Autodesk Inventor part; units mm, degrees
ref_plane "YZ Plane" through (0, 0, 0) normal (1, 0, 0) x (0, 1, 0)
ref_plane "XZ Plane" through (0, 0, 0) normal (0, 1, 0) x (-1, 0, 0)
ref_plane "XY Plane" through (0, 0, 0) normal (0, 0, 1) x (1, 0, 0)
sketch "Sketch1" plane through (0, 0, 0) normal (1, 0, 0) x (0, 1, 0)
  line L0 (11, 31.5) -> (-11, 31.5)
  line L1 (-11, 31.5) -> (-11, -31.5)
  line L2 (-11, -31.5) -> (11, -31.5)
  line L3 (11, -31.5) -> (11, 31.5)
  line L4 (11, 31.5) -> (-11, -31.5) construction
  line L5 (-11, 31.5) -> (11, -31.5) construction
  point P0 (0, 0)
  dimension "d0" = 22
  dimension "d1" = 63
extrude "Extrusion1" add sketch "Sketch1" along normal mid plane 141
fillet "Fillet1" radius 6 4 edges at (0, 11, 31.5) (0, 11, -31.5) (0, -11, 31.5) (0, -11, -31.5)
sketch "Sketch2" plane through (70.5, 0, 0) normal (1, 0, 0) x (0, 0, -1)
  line L0 (10.5, 7) -> (24.5, 7)
  line L1 (24.5, 7) -> (24.5, 1)
  line L2 (24.5, 1) -> (10.5, 1)
  line L3 (10.5, 1) -> (10.5, 7)
  line L4 (31.5, -5) -> (31.5, 5)
  line L5 (25.5, 11) -> (-25.5, 11)
  line L6 (11.7, 5.85) -> (23.3, 5.85)
  line L7 (23.3, 5.85) -> (23.3, 4.6)
  line L8 (23.3, 4.6) -> (11.7, 4.6)
  line L9 (11.7, 4.6) -> (11.7, 5.85)
  line L10 (10.5, -2.5) -> (24.5, -2.5)
  line L11 (24.5, -2.5) -> (24.5, -8.5)
  line L12 (24.5, -8.5) -> (10.5, -8.5)
  line L13 (10.5, -8.5) -> (10.5, -2.5)
  line L14 (11.7, -3.65) -> (23.3, -3.65)
  line L15 (23.3, -3.65) -> (23.3, -4.9)
  line L16 (23.3, -4.9) -> (11.7, -4.9)
  line L17 (11.7, -4.9) -> (11.7, -3.65)
  point P0 (0, 0)
  dimension "d5" = 14
  dimension "d6" = 6
  dimension "d7" = 7
  dimension "d8" = 4
  dimension "d12" = 1.2
  dimension "d13" = 1.2
  dimension "d14" = 1.15
  dimension "d15" = 3.6
  dimension "d16" = 14
  dimension "d17" = 6
  dimension "d18" = 1.2
  dimension "d19" = 1.2
  dimension "d20" = 1.15
  dimension "d21" = 3.6
  dimension "d22" = 3.5
extrude "Extrusion2" cut sketch "Sketch2" against normal blind 10
sketch "Sketch3" plane through (-70.5, 11, -25.5) normal (0, 1, 0) x (1, 0, 0)
  line L0 (110.1613, -6.5149) -> (123.1613, -6.5149)
  line L1 (123.1613, -6.5149) -> (123.1613, -10.5149)
  line L2 (123.1613, -10.5149) -> (110.1613, -10.5149)
  line L3 (110.1613, -10.5149) -> (110.1613, -6.5149)
  line L4 (110.6613, -7.0149) -> (112.6613, -7.0149)
  line L5 (112.6613, -7.0149) -> (112.6613, -10.0149)
  line L6 (112.6613, -10.0149) -> (110.6613, -10.0149)
  line L7 (110.6613, -10.0149) -> (110.6613, -7.0149)
  line L8 (115.9613, -10.0149) -> (113.9613, -10.0149)
  line L9 (113.9613, -10.0149) -> (113.9613, -7.0149)
  line L10 (113.9613, -7.0149) -> (115.9613, -7.0149)
  line L11 (115.9613, -7.0149) -> (115.9613, -10.0149)
  line L12 (119.2613, -10.0149) -> (117.2613, -10.0149)
  line L13 (117.2613, -10.0149) -> (117.2613, -7.0149)
  line L14 (117.2613, -7.0149) -> (119.2613, -7.0149)
  line L15 (119.2613, -7.0149) -> (119.2613, -10.0149)
  line L16 (122.5613, -10.0149) -> (120.5613, -10.0149)
  line L17 (120.5613, -10.0149) -> (120.5613, -7.0149)
  line L18 (120.5613, -7.0149) -> (122.5613, -7.0149)
  line L19 (122.5613, -7.0149) -> (122.5613, -10.0149)
  point P0 (70.5, -25.5)
  dimension "d25" = 13
  dimension "d26" = 4
  dimension "d27" = 2
  dimension "d28" = 3
  dimension "d29" = 0.5
  dimension "d30" = 0.5
  dimension "d33" = 3.3
extrude "Extrusion3" cut sketch "Sketch3" against normal blind 0.25
sketch "Sketch4" plane through (70.5, -5, -31.5) normal (0, 0, -1) x (-1, 0, 0)
  line L0 (141, 10) -> (0, 10) construction
  line L1 (0, 0) -> (0, 10) construction
  line L2 (35, 5) -> (42, 5)
  line L3 (42, 5) -> (42, 8)
  line L4 (42, 8) -> (35, 8)
  line L5 (35, 8) -> (35, 5)
  line L6 (38.5, 5) -> (38.5, 8) construction
  line L7 (35, 6.5) -> (36.7876, 5)
  line L8 (35, 6.5) -> (37.3336, 6.5) construction
  line L9 (42, 6.5) -> (40.2124, 5)
  line L10 (42, 6.5) -> (42, 5)
  line L11 (40.2124, 5) -> (42, 5)
  point P0 (70.5, 5)
  dimension "d42" = 3
  dimension "d43" = 35
  dimension "d44" = 7
  dimension "d45" = 2
  dimension "d46" = 40
extrude "Extrusion4" cut sketch "Sketch4" against normal blind 5 contours L7 L5 L4 L3 L9 L2
sketch "Sketch5" plane through (70.5, -5, -31.5) normal (0, 0, -1) x (-1, 0, 0)
  line L0 (0, 0) -> (0, 10) construction
  line L1 (0, 5) -> (141, 5) construction
  line L2 (141, 10) -> (141, 0) construction
  line L3 (13, 9) -> (27, 9)
  line L4 (27, 9) -> (27, 1)
  line L5 (27, 1) -> (13, 1)
  line L6 (13, 1) -> (13, 9)
  line L7 (13, 9) -> (27, 1) construction
  line L8 (27, 9) -> (13, 1) construction
  line L9 (26.75, 8.75) -> (13.25, 8.75)
  line L10 (13.25, 8.75) -> (13.25, 1.25)
  line L11 (13.25, 1.25) -> (26.75, 1.25)
  line L12 (26.75, 1.25) -> (26.75, 8.75)
  line L13 (35, 6.5) -> (35, 8)
  point P0 (70.5, 5)
  point P1 (20, 5)
  dimension "d49" = 14
  dimension "d50" = 8
  dimension "d51" = 0.25
  dimension "d52" = 8
extrude "Extrusion5" cut sketch "Sketch5" against normal blind 0.1
sketch "Sketch6" plane through (70.5, 0, 0) normal (1, 0, 0) x (0, 0, -1)
  line L0 (10.5, 1) -> (10.5, 7)
  line L1 (10.5, 7) -> (24.5, 7)
  line L2 (24.5, 7) -> (24.5, 1)
  line L3 (24.5, 1) -> (10.5, 1)
  line L4 (10.5, -8.5) -> (10.5, -2.5)
  line L5 (10.5, -2.5) -> (24.5, -2.5)
  line L6 (24.5, -2.5) -> (24.5, -8.5)
  line L7 (24.5, -8.5) -> (10.5, -8.5)
  arc A0 (25.5, -11) -> (31.5, -5) centre (25.5, -5) ccw
  line L8 (31.5, -5) -> (31.5, 5)
  arc A1 (31.5, 5) -> (25.5, 11) centre (25.5, 5) ccw
  line L9 (25.5, 11) -> (-25.5, 11)
  arc A2 (-25.5, 11) -> (-31.5, 5) centre (-25.5, 5) ccw
  line L10 (-31.5, 5) -> (-31.5, -5)
  arc A3 (-31.5, -5) -> (-25.5, -11) centre (-25.5, -5) ccw
  line L11 (-25.5, -11) -> (25.5, -11)
  line L12 (-25.5, 10) -> (25.5, 10)
  arc A4 (30.5, 5) -> (25.5, 10) centre (25.5, 5) ccw
  line L13 (30.5, 5) -> (30.5, -5)
  arc A5 (25.5, -10) -> (30.5, -5) centre (25.5, -5) ccw
  line L14 (25.5, -10) -> (-25.5, -10)
  arc A6 (-30.5, -5) -> (-25.5, -10) centre (-25.5, -5) ccw
  line L15 (-30.5, -5) -> (-30.5, 5)
  arc A7 (-25.5, 10) -> (-30.5, 5) centre (-25.5, 5) ccw
  line L16 (-25.5, 9.75) -> (25.5, 9.75)
  arc A8 (30.25, 5) -> (25.5, 9.75) centre (25.5, 5) ccw
  line L17 (30.25, 5) -> (30.25, -5)
  arc A9 (25.5, -9.75) -> (30.25, -5) centre (25.5, -5) ccw
  line L18 (25.5, -9.75) -> (-25.5, -9.75)
  arc A10 (-30.25, -5) -> (-25.5, -9.75) centre (-25.5, -5) ccw
  line L19 (-30.25, -5) -> (-30.25, 5)
  arc A11 (-25.5, 9.75) -> (-30.25, 5) centre (-25.5, 5) ccw
  point P0 (0, 0)
  dimension "d55" = 1
  dimension "d56" = 1.25
extrude "Extrusion6" cut sketch "Sketch6" against normal blind 0.1 contours L12 A4 L13 A5 L14 A6 L15 A7
mirror "Mirror1" about plane through (0, 0, 0) normal (1, 0, 0) of "Extrusion6"
properties part number "Battery"
Design review of the part built by this model. Coordinates are the model's own, in mm. A direction names the side the tool comes from. Give positions to 0.01 mm unless a question says otherwise; leave off trailing zeros. Order: outer loops, then holes, each group sorted by start corner. A loop starts at its lowest first (then second) coordinate and runs counter-clockwise, first axis right, second up. Notation, with made-up numbers: (-28, 57) -> (27, 57) arc R19 cw to (27, 67) -> close; hole circle Ø7 at (-29, 19). An arc over 180 degrees is marked (long way). Write item = value, one per line. Start each with the question number.
(1) To check wall thickness, follow line 1 along X through (y, z) = (-7.5, -13); line 2 along Y through (x, z) = (-39, 28); line 3 along Z through (x, y) = (57.5, 8.75). State the ranges of each line that lie inside material, in increasing order.
(2) We need section B-B on y = 8.5. Write out the cut boundary in (x, z), plus the area to 3 significant figures.
(3) For faces 4 (the face through (66, -2.5, -17)), 5 (the face through (50, 0, -31.5)), list the 3-axis set-ups (+Z, -Z, +X, -X, +Y, -Y) from which the entire face can be reached by the end or side of a thin tool; tool diameter is ignored.
(4) We need section A-A on x = -25. Write out the cut boundary in (y, z).
(5) Mouldability with a two-part tool opening along Z and no side actions: class faces 1 (the face through (66, 4.6, -18)), 2 (the face through (32, 2, -26.5)), 3 (the face through (70.5, 0, 0)) as +Z half, -Z half, draft (parallel to the pull), parting line (faces both ways), or undercut.
(6) For pin 1 (3.5 mm diameter, centred on x = 30.5, y = 1.5, fed in from -Z); pin 2 (5.5 mm diameter, centred on x = 32, z = -29, fed in from -Y), all flat-tipped, find the tip position at first contact; note any pin that passes through.
Numbers:
q1.line_1 = -70.5 to 60.5
q1.line_2 = -10.45 to 10.45
q1.line_3 = -30.18 to 30.18
q2.outline = (-70.5, -30.37) -> (70.5, -30.37) -> (70.5, -29.07) -> (70.4, -29.07) -> (70.4, -28.71) -> (70.5, -28.71) -> (70.5, 28.71) -> (70.4, 28.71) -> (70.4, 29.07) -> (70.5, 29.07) -> (70.5, 30.37) -> (-70.5, 30.37) -> (-70.5, 29.07) -> (-70.4, 29.07) -> (-70.4, 28.71) -> (-70.5, 28.71) -> (-70.5, -28.71) -> (-70.4, -28.71) -> (-70.4, -29.07) -> (-70.5, -29.07) -> close
q2.area = 8,570 mm^2
q3.face_4 = +X
q3.face_5 = -Z, +X, -X, +Y, -Y
q4.outline = (-11, -25.5) arc R6 ccw to (-5, -31.5) -> (5, -31.5) arc R6 ccw to (11, -25.5) -> (11, 25.5) arc R6 ccw to (5, 31.5) -> (-5, 31.5) arc R6 ccw to (-11, 25.5) -> close
q5.face_1 = undercut
q5.face_2 = -Z half
q5.face_3 = draft
q6.pin_1 = -31.5
q6.pin_2 = -10.95
